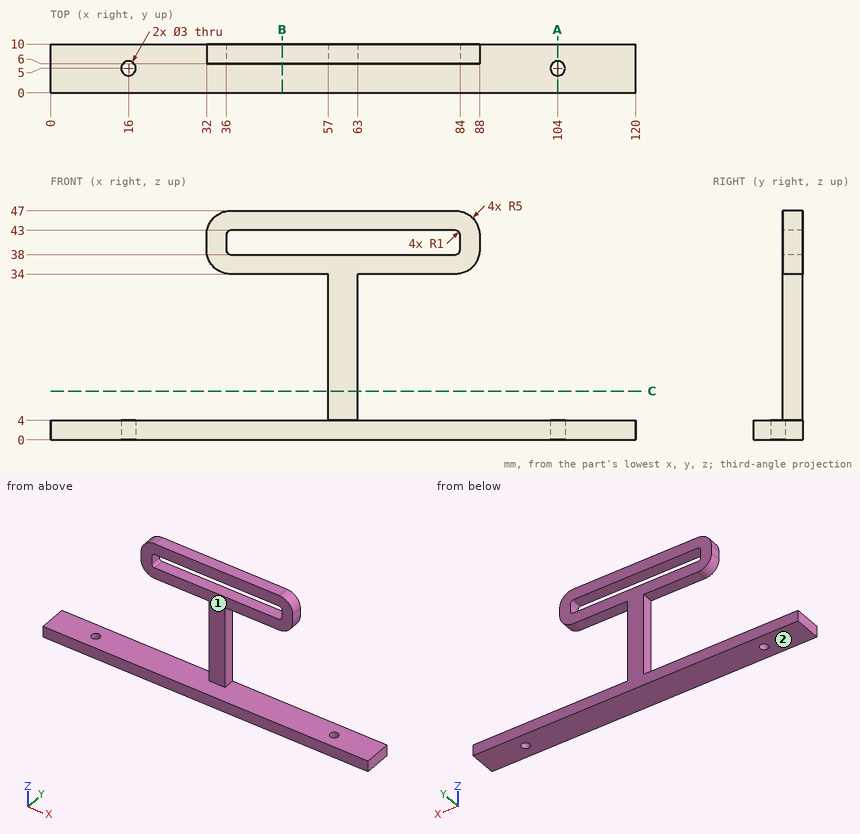
Check sheet for the drawn part. Datum: minimum x, y, z corner. Units: mm. A direction names the side the tool comes from. Round coordinates to 2 decimals unless told otherwise and drop trailing zeros. Order: outer loops, then holes, each group sorted by start corner. A loop starts at its lowest first (then second) coordinate and runs counter-clockwise, first axis right, second up.
(1) Cross-section at A-A, the plane x = 104. Enter the section's corners in (y, z).
(2) Scan lines: probe 1 along Z at (x, y) = (42, 8.75); probe 2 along Y at (x, z) = (16, 1.6); probe 3 along X at (y, z) = (6, 2.5). Record each from-to range of solid material in increasing order.
(3) Cross-section at C-C, the plane z = 10. Enter the section's corners in (x, y).
(4) Access from +Z, -Z, +X, -X, +Y, -Y to the whole of each face (thin tool, end or side, straight path). Record for the marked faces 1 and 2.
(5) Go/stop test with flat-tipped pins: P1, Ø4.5, axis at y = 8, z = 19, coming from the -X side; P2, Ø2.5, axis at y = 8.5, z = 40, coming from the -X side; P3, Ø3.5, axis at x = 104, y = 5, coming from the +Z side. Record where each tip stops, or that it passes through.
(6) Cross-section at B-B, the plane x = 47.5. Enter the section's corners in (y, z), and give its area (3 significant figures).
Check sheet entries:
1. outline: (0, 0) - (3.5, 0) - (3.5, 4) - (0, 4) - close; (6.5, 0) - (10, 0) - (10, 4) - (6.5, 4) - close
2. probe 1: z = 0 to 4, 34 to 38, 43 to 47
2. probe 2: y = 0 to 3.5, 6.5 to 10
2. probe 3: x = 0 to 14.88, 17.12 to 102.88, 105.12 to 120
3. outline: (57, 6) - (63, 6) - (63, 10) - (57, 10) - close
4. face 1: +Z, +X, -X, -Y
4. face 2: -Z, +X, -X, +Y, -Y
5. P1: stops at x = 57
5. P2: stops at x = 32
5. P3: stops at z = 4
6. outline: (0, 0) - (10, 0) - (10, 4) - (0, 4) - close; (6, 34) - (10, 34) - (10, 38) - (6, 38) - close; (6, 43) - (10, 43) - (10, 47) - (6, 47) - close
6. area: 72.0 mm2
